The listing builds one solid part. Answer for the finished solid, in the listing's coordinates (mm). Face numbers are marked on the shaded views. Coordinates: 2 decimals unless noted, no trailing zeros. Order: outer loops, then holes, each group sorted by start corner. A loop starts at its lowest first (then second) coordinate and runs counter-clockwise, first axis right, second up.
from build123d import *

# Parameters (mm, degrees)
SKETCH1_W           = 29
SKETCH1_H           = 12.7
BOSS_EXTRUDE1_DEPTH = 15.7
BOSS_EXTRUDE1_DRAFT = 0.05
CUT_EXTRUDE1_DEPTH  = 0.2
SKETCH3_W           = 0.4
SKETCH3_H           = 0.6
SKETCH3_W_2         = 0.5
SKETCH3_H_2         = 0.8
BOSS_EXTRUDE2_DEPTH = 3.8
FILLET1_R           = 0.3
FILLET2_R           = 0.4
SKETCH4_W           = 3.182056495
SKETCH4_H           = 2.2
SKETCH4_R           = 0.5
CUT_EXTRUDE2_DEPTH  = 1
FILLET3_R           = 0.1


with BuildPart() as part:
    # Sketch1 → Boss-Extrude1 (with draft: the straight prism first)
    with BuildSketch(Plane(origin=(0, 0, 0), x_dir=(1, 0, 0), z_dir=(0, 1, 0))):
        Rectangle(SKETCH1_W, SKETCH1_H)
    extrude(amount=-BOSS_EXTRUDE1_DEPTH)
    # Boss-Extrude1: the draft: its side faces are tilted about the plane it starts from
    boss_extrude1_sides = [part.faces().sort_by_distance(p)[0] for p in [
        (-14.5, -7.85, 0),
        (0, -7.85, 6.35),
        (14.5, -7.85, 0),
        (0, -7.85, -6.35),
    ]]
    draft(boss_extrude1_sides, Plane(origin=(0, 0, 0), x_dir=(1, 0, 0), z_dir=(0, 1, 0)), BOSS_EXTRUDE1_DRAFT)

    # Sketch2 → Cut-Extrude1 (cut)
    with BuildSketch(Plane(origin=(0, -15.7, 0), x_dir=(-1, 0, 0), z_dir=(0, -1, 0))):
        Polygon((14.013700838, -5.863700838), (12.513700838, -5.863700838), (12.513700838, -6.363700838), (-12.513700838, -6.363700838), (-12.513700838, -5.863700838), (-14.013700838, -5.863700838), (-14.013700838, -4.463700838), (-14.513700838, -4.463700838), (-14.513700838, 4.463700838), (-14.013700838, 4.463700838), (-14.013700838, 5.863700838), (-12.513700838, 5.863700838), (-12.513700838, 6.363700838), (12.513700838, 6.363700838), (12.513700838, 5.863700838), (14.013700838, 5.863700838), (14.013700838, 4.463700838), (14.513700838, 4.463700838), (14.513700838, -4.463700838), (14.013700838, -4.463700838), align=None)
    extrude(amount=-CUT_EXTRUDE1_DEPTH, mode=Mode.SUBTRACT)

    # Sketch3 → Boss-Extrude2 (add)
    with BuildSketch(Plane.XZ.offset(15.5)):
        with Locations((11.786299162, -3.8)):
            Rectangle(SKETCH3_W, SKETCH3_H)
        with Locations((11.786299162, 3.8)):
            Rectangle(SKETCH3_W, SKETCH3_H)
        with Locations((-8.213700838, 3.8)):
            Rectangle(SKETCH3_W_2, SKETCH3_H_2)
        with Locations((-13.213700838, -3.8)):
            Rectangle(SKETCH3_W_2, SKETCH3_H_2)
        with Locations((-13.213700838, 3.8)):
            Rectangle(SKETCH3_W_2, SKETCH3_H_2)
        with Locations((-8.213700838, -3.8)):
            Rectangle(SKETCH3_W_2, SKETCH3_H_2)
        with Locations((-3.213700838, 3.8)):
            Rectangle(SKETCH3_W_2, SKETCH3_H_2)
        with Locations((-3.213700838, -3.8)):
            Rectangle(SKETCH3_W_2, SKETCH3_H_2)
    extrude(amount=BOSS_EXTRUDE2_DEPTH)

    # Fillet1
    fillet1_edges = [part.edges().sort_by_distance(p)[0] for p in [
        (11.786299162, -19.3, 4.1),
        (11.786299162, -19.3, 3.5),
        (11.786299162, -19.3, -3.5),
        (11.786299162, -19.3, -4.1),
    ]]
    fillet(fillet1_edges, radius=FILLET1_R - 0.0001)  # a hair under: the kernel refuses the full size

    # Fillet2
    fillet2_edges = [part.edges().sort_by_distance(p)[0] for p in [
        (-13.213700838, -19.3, -4.2),
        (-13.213700838, -19.3, -3.4),
        (-8.213700838, -19.3, 4.2),
        (-8.213700838, -19.3, 3.4),
        (-13.213700838, -19.3, 3.4),
        (-13.213700838, -19.3, 4.2),
        (-8.213700838, -19.3, -4.2),
        (-8.213700838, -19.3, -3.4),
        (-3.213700838, -19.3, -4.2),
        (-3.213700838, -19.3, -3.4),
        (-3.213700838, -19.3, 3.4),
        (-3.213700838, -19.3, 4.2),
    ]]
    fillet(fillet2_edges, radius=FILLET2_R - 0.0001)  # a hair under: the kernel refuses the full size

    # Sketch4 → Cut-Extrude2 (cut)
    with BuildSketch(Plane(origin=(0, 0, 0), x_dir=(1, 0, 0), z_dir=(0, 1, 0))):
        with Locations((13.891028247, 0)):
            Rectangle(SKETCH4_W, SKETCH4_H)
        with Locations(Location((13.4, 0, 0), (0, 0, 270))):
            Circle(SKETCH4_R, mode=Mode.SUBTRACT)
    extrude(amount=-CUT_EXTRUDE2_DEPTH, mode=Mode.SUBTRACT)

    # Fillet3
    fillet3_edges = [part.edges().sort_by_distance(p)[0] for p in [
        (14.5, 0, -3.725),
        (13.4, 0, -1.1),
        (14.500872665, -1, 0),
        (14.500436332, -0.5, -1.1),
        (14.500436332, -0.5, 1.1),
        (13.4, 0, 1.1),
        (12.3, 0, 0),
        (13.4, 0, -0.5),
        (0, 0, 6.35),
        (-14.5, 0, 0),
        (0, 0, -6.35),
        (14.5, 0, 3.725),
        (14.506850419, -7.85, 6.356850419),
        (-14.506850419, -7.85, 6.356850419),
        (-14.506850419, -7.85, -6.356850419),
        (14.506850419, -7.85, -6.356850419),
    ]]
    fillet(fillet3_edges, radius=FILLET3_R)


solid = part.part
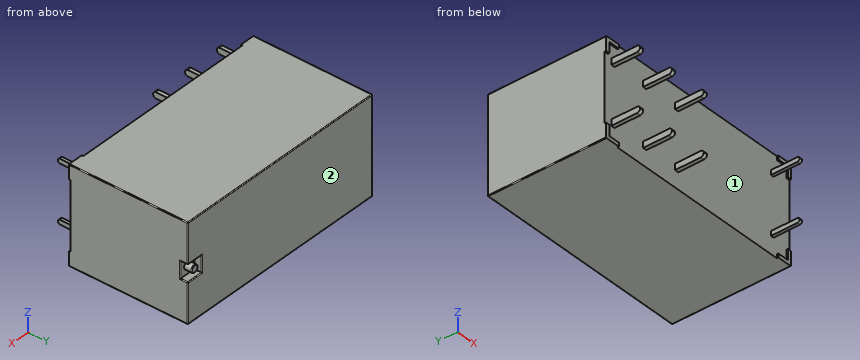
(1) Find the intervals of material crossed by probe 1 along Z at (x, y) = (9, -3.5); probe 2 along Y at (x, z) = (-2.75, 2.25); probe 3 along X at (y, z) = (-6.25, 3.25), in increasing order.
(2) The mould has two halves that part along X. Classify the marked faces 1 and 2: pulls with the +X half, pulls with the -X half, needs draft (parallel to the pull), parting line crosses it, or undercut.
(3) Find section C-C on x = -5. Determine the outline of the cut face in (y, z).
(4) Find section D-D on z = -3. Determine the outline of the cut face in (x, y), then the cut area to 3 significant figures.
(5) Find section B-B on z = 0. Determine the outline of the cut face in (x, y).
(6) Given pin 1 Ø0.9 at (y, z) = (-17, 3.5) entering from +X; pin 2 Ø10 at (x, y) = (-4.5, -2) entering from -Z; pin 3 Ø0.6 at (y, z) = (-17, -3.5) entering from -X, each flat-ended and moving along its own axis, determine where each tip first touches the part or whether it passes through.
(7) Find section A-A on x = 13.4. Determine the outline of the cut face in (y, z).
Resolved:
1. probe 1: z = -6.35 to 6.35
1. probe 2: y = -15.5 to 0
1. probe 3: x = -14.51 to 14.51
2. face 1: undercut
2. face 2: needs draft
3. outline: (-15.5, -6.36) - (-0.1, -6.35) arc R0.1 ccw to (0, -6.25) - (0, 6.25) arc R0.1 ccw to (-0.1, 6.35) - (-15.5, 6.36) - close
4. outline: (-14.51, -15.5) - (14.51, -15.5) - (14.5, -0.1) arc R0.1 ccw to (14.4, 0) - (-14.4, 0) arc R0.1 ccw to (-14.5, -0.1) - close
4. area: 450 mm2
5. outline: (-14.51, -15.5) - (14.51, -15.5) - (14.5, -1.1) arc R0.1 ccw to (14.4, -1) - (13.9, -1) - (13.9, -0.1) arc R0.1 ccw to (13.8, 0) - (13, 0) arc R0.1 ccw to (12.9, -0.1) - (12.9, -1) - (12.3, -1) - (12.3, -0.1) arc R0.1 ccw to (12.2, 0) - (-14.4, 0) arc R0.1 ccw to (-14.5, -0.1) - close
6. pin 1: stops at x = 11.99
6. pin 2: stops at z = -6.36
6. pin 3: stops at x = -13.46
7. outline: (-15.7, -6.36) - (-0.1, -6.35) arc R0.1 ccw to (0, -6.25) - (0, -1.2) arc R0.1 ccw to (-0.1, -1.1) - (-1, -1.1) - (-1, -0.5) - (-0.1, -0.5) arc R0.1 ccw to (0, -0.4) - (0, 0.4) arc R0.1 ccw to (-0.1, 0.5) - (-1, 0.5) - (-1, 1.1) - (-0.1, 1.1) arc R0.1 ccw to (0, 1.2) - (0, 6.25) arc R0.1 ccw to (-0.1, 6.35) - (-15.7, 6.36) - (-15.7, 5.86) - (-15.5, 5.86) - (-15.5, -5.86) - (-15.7, -5.86) - close
